Read the model definition and answer for the solid it produces. Units are mm, in the model's axes. A direction names the side the tool comes from. Coordinates: 2 decimals unless noted, no trailing zeros. Write each loop counter-clockwise with the first axis right and the second up, starting at its lowest first coordinate (ties: lowest second). Pieces come first, ordered by that corner, then holes. Notation, with made-up numbers: (25.25, 4.5) -> (47.25, 4.5) arc R16 cw to (47.25, 15.5) -> close; hole circle Ø4 at (82, -11). An arc over 180 degrees is marked (long way). Write item = value, one per line. Start each with the question number.
1) Section B-B (z = 3.25) is taken. Determine the outline of the cut face in (x, y).
2) Flat-ended cylindrical pins translate along their axes: pin 1 Ø8 at (x, y) = (11, 24) entering from -Z; pin 2 Ø1.1 at (y, z) = (9, 3.5) entering from -X; pin 3 Ø0.8 at (x, z) = (0.5, 4) entering from +Y. Find the tip coordinate at first contact, or state that the pin passes through.
3) Section A-A (y = 20.5) is taken. Determine the outline of the cut face in (x, z), plus the area to 3 significant figures.
4) Find the intervals of material crossed by line 1 along Z through (x, y) = (-7, 6); line 2 along X through (y, z) = (18, 5.1), in increasing order. Write a range as from..to.
5) A tool of negligible diameter and unlimited length cuts with its end or side. For faces 1 (the face through (0, 16, 4)), 2 (the face through (0.5, 29, 4.1)), 3 (the face through (0.5, 2, 4.1)), from which of +Z, -Z, +X, -X, +Y, -Y can it reach the whole face along a straight path? Write none if from no direction.
6) Section C-C (x = -12) is taken. Determine the outline of the cut face in (y, z), plus the area to 3 significant figures.
from build123d import *

# Parameters (mm, degrees)
SKETCH_W        = 42.5
SKETCH_H        = 36
PAD_DEPTH       = 6
SKETCH001_W     = 38.5
SKETCH001_H     = 32
POCKET_DEPTH    = 5
SKETCH002_W     = 40.5
SKETCH002_H     = 34
POCKET001_DEPTH = 1.2
SKETCH003_W     = 1
SKETCH003_H     = 27
PAD001_DEPTH    = 3.8
SKETCH004_W     = 40.5
SKETCH004_H     = 34
PAD002_DEPTH    = 2
SKETCH005_W     = 42.5
SKETCH005_H     = 6
POCKET002_DEPTH = 36.001
SKETCH006_W     = 1
SKETCH006_H     = 27
PAD003_DEPTH    = 3.8


with BuildPart() as part:
    # Sketch → Pad (new body)
    with BuildSketch(Plane.XY):
        with Locations((0.25, 18)):
            Rectangle(SKETCH_W, SKETCH_H)
    extrude(amount=PAD_DEPTH)

    # Sketch001 (on Face6 of Pad) → Pocket (cut)
    with BuildSketch(Plane.XY.offset(6)):
        with Locations((0.25, 18)):
            Rectangle(SKETCH001_W, SKETCH001_H)
    extrude(amount=-POCKET_DEPTH, mode=Mode.SUBTRACT)

    # Sketch002 (on Face5 of Pocket) → Pocket001 (cut)
    with BuildSketch(Plane.XY.offset(6)):
        with Locations((0.25, 18)):
            Rectangle(SKETCH002_W, SKETCH002_H)
    extrude(amount=-POCKET001_DEPTH, mode=Mode.SUBTRACT)

    # Sketch003 (on Face16 of Pocket001) → Pad001 (join)
    with BuildSketch(Plane.XY.offset(1)):
        with Locations((-0.5, 20.5)):
            Rectangle(SKETCH003_W, SKETCH003_H)
    extrude(amount=PAD001_DEPTH)

    # Sketch004 (on Face11 of Pad001) → Pad002 (join)
    with BuildSketch(Plane.XY.offset(4.8)):
        with Locations((0.25, 18)):
            Rectangle(SKETCH004_W, SKETCH004_H)
    extrude(amount=PAD002_DEPTH)

    # Sketch005 (on Face1 of Pad002) → Pocket002 (cut, through all)
    with BuildSketch(Plane.XZ):
        with Locations((0.25, 3)):
            Rectangle(SKETCH005_W, SKETCH005_H)
    extrude(amount=-POCKET002_DEPTH, mode=Mode.SUBTRACT)

    # Sketch006 (on Face2 of Pocket002) → Pad003 (join)
    with BuildSketch(Plane(origin=(0, 0, 6), x_dir=(1, 0, 0), z_dir=(0, 0, -1))):
        with Locations((0.5, -15.5)):
            Rectangle(SKETCH006_W, SKETCH006_H)
    extrude(amount=PAD003_DEPTH)


solid = part.part
Answer key:
q1.outline = (0, 2) -> (1, 2) -> (1, 29) -> (0, 29) -> close
q2.pin_1 = 6
q2.pin_2 = 0
q2.pin_3 = 29
q3.outline = (-20, 6) -> (0, 6) -> (0, 2.2) -> (1, 2.2) -> (1, 6) -> (20.5, 6) -> (20.5, 6.8) -> (-20, 6.8) -> close
q3.area = 36.2 mm^2
q4.line_1 = 6..6.8
q4.line_2 = 0..1
q5.face_1 = -Z, -X, +Y, -Y
q5.face_2 = -Z, +X, -X, +Y
q5.face_3 = -Z, +X, -X, -Y
q6.outline = (1, 6) -> (35, 6) -> (35, 6.8) -> (1, 6.8) -> close
q6.area = 27.2 mm^2
